from build123d import *

# Parameters (mm, degrees)
F1_DEPTH = 2409
F3_DEPTH = 100
F5_DEPTH = 100


with BuildPart() as f1:
    # F0 (on Front) → F1 (new body)
    with BuildSketch(Plane.XZ):
        Polygon((-90, -90), (90, -90), (90, -75), (10, -75), (10, 75), (90, 75), (90, 90), (-90, 90), (-90, 75), (-10, 75), (-10, -75), (-90, -75), align=None)
    extrude(amount=-F1_DEPTH)

    # F2 (on Front) → F3 (join)
    with BuildSketch(Plane.XZ):
        Polygon((90, -274.244994), (90, -90), (-90, -90), (-90, -274.244994), (-90, -910), (90, -910), align=None)
        Polygon((590, -910), (90, -90), (90, -274.244994), (477.655492, -910), align=None)
        Polygon((-90, -274.244994), (-90, -90), (-590, -910), (-477.655492, -910), align=None)
    extrude(amount=-F3_DEPTH)

    # F4 (on face) → F5 (join)
    with BuildSketch(Plane(origin=(0, 2409, 0), x_dir=(-1, 0, 0), z_dir=(0, 1, 0))):
        Polygon((90, -910), (90, -274.244994), (477.655492, -910), (590, -910), (90, -90), (-90, -90), (-590, -910), (-477.655492, -910), (-90, -274.244994), (-90, -910), align=None)
    extrude(amount=-F5_DEPTH)


solid = f1.part
Verification items for the finished model (mm, model axes). A direction names the side the tool comes from. Coordinates: 2 decimals unless noted, no trailing zeros. Loops run counter-clockwise (first coordinate to the right, second up) from the corner with the lowest first, then second, coordinate; pieces in that order, holes last. Notation, with made-up numbers: M 76.5,10 L 98.5,10 A8 cw 98.5,24 Z; hole C 86,16.25 d8. An arc over 180 degrees is marked long. One line per item, written item: value.
1. Section check A-A on x = 63. Record the cut outline in (y, z), plus the area to 3 significant figures.
Answers follow:
outline: M 0,-910 L 100,-910 L 100,-90 L 2309,-90 L 2309,-910 L 2409,-910 L 2409,-75 L 0,-75 Z; M 0,75 L 2409,75 L 2409,90 L 0,90 Z
area: 236,000 mm^2
2. Section check D-D on x = -196. Record the cut outline in (y, z) (3 decimals).
Answers follow:
outline: M 0,-448.085 L 100,-448.085 L 100,-263.84 L 0,-263.84 Z; M 2309,-448.085 L 2409,-448.085 L 2409,-263.84 L 2309,-263.84 Z
3. Section check C-C on y = 1133. Record the cut outline in (x, z), plus the area to 3 significant figures.
Answers follow:
outline: M -90,-90 L 90,-90 L 90,-75 L 10,-75 L 10,75 L 90,75 L 90,90 L -90,90 L -90,75 L -10,75 L -10,-75 L -90,-75 Z
area: 8,400 mm^2
4. Material ranges on line 1 along Y through (x, z) = (-47, -615); line 2 along Z through (x, y) = (16.5, 350.5); line 3 along X through (y, z) = (879, -52), recorded low to high. Write a range as from..to.
Answers follow:
line 1: 0..100, 2309..2409
line 2: -90..-75, 75..90
line 3: -10..10
5. Gauge pin test, flat ends, axial feed: P1, Ø12, axis at y = 1277, z = 81, coming from the -X side; P2, Ø12, axis at y = 859, z = 81, coming from the +X side. Record the tip position at first contact, or that the pin passes through.
Answers follow:
P1: x = -90
P2: x = 90
6. Set-up check for faces 1 (the flat face through (3, 2309, -528)), 2 (the flat face through (-281.114, 2359.7, -587.672)), 3 (the flat face through (-51, 1188, 75)): record each of +Z, -Z, +X, -X, +Y, -Y from which the full face is reachable in a straight line by a thin tool's end or side.
Answers follow:
face 1: -Z, +X, -X
face 2: -Z, +Y, -Y
face 3: -X, +Y, -Y
7. Mould release check, pull along Z, two halves, no side actions. Record for faces 4 (the flat face through (49, 1188, 75)), 5 (the flat face through (1, 2360, -910)), 6 (the flat face through (-3, 100, -528)): pulls with the +Z half, pulls with the -Z half, needs draft (parallel to the pull), parting line crosses it, or undercut.
Answers follow:
face 4: undercut
face 5: pulls with the -Z half
face 6: needs draft
8. Section check B-B on z = -114.5. Record the cut outline in (x, y), plus the area to 3 significant figures.
Answers follow:
outline: M -104.94,0 L 104.94,0 L 104.94,100 L -104.94,100 Z; M -104.94,2309 L 104.94,2309 L 104.94,2409 L -104.94,2409 Z
area: 42,000 mm^2
